```python
from build123d import *

# Parameters (mm, degrees)
CROQUIS1_R              = 1.5
SALIENTE_EXTRUIR1_DEPTH = 9


with BuildPart() as part:
    # Croquis1 → Saliente-Extruir1 (new body)
    with BuildSketch(Plane(origin=(0, 0, 0), x_dir=(1, 0, 0), z_dir=(0, 1, 0))):
        Polygon((7.75, 7.5), (26.5, 22.904273087), (26.5, 77.904273087), (26.5, 87.904273087), (41.5, 77.904273087), (41.5, 22.904273087), (22.75, 7.5), (22.75, -7.5), (7.75, -7.5), align=None)
        with Locations(Location((19.25, 4, 0), (0, 0, 270))):
            Circle(CROQUIS1_R, mode=Mode.SUBTRACT)
        with Locations(Location((19.25, -4, 0), (0, 0, 270))):
            Circle(CROQUIS1_R, mode=Mode.SUBTRACT)
        with Locations(Location((11.25, -4, 0), (0, 0, 270))):
            Circle(CROQUIS1_R, mode=Mode.SUBTRACT)
        with Locations(Location((11.25, 4, 0), (0, 0, 270))):
            Circle(CROQUIS1_R, mode=Mode.SUBTRACT)
    extrude(amount=SALIENTE_EXTRUIR1_DEPTH)


solid = part.part
```
Here's how the part is built. I have some questions about the finished solid (model axes, mm). A direction names the side the tool comes from. Round coordinates to 2 decimals unless told otherwise and drop trailing zeros. Order: outer loops, then holes, each group sorted by start corner. A loop starts at its lowest first (then second) coordinate and runs counter-clockwise, first axis right, second up. Notation, with made-up numbers: (10.25, 69.25) -> (49.25, 69.25) arc R21 ccw to (49.25, 75.25) -> close; hole circle Ø6 at (59, -11). An arc over 180 degrees is marked (long way). Use a Markdown table: item, result. Add a question column.
(1) I need wall thicknesses on line 1 along X through (y, z) = (4, -4); line 2 along Z through (x, y) = (20, 2.25); line 3 along X through (y, z) = (2, -71). Which ranges of each line are inside material? Lowest first, please.
(2) For faces 1 (the face through (41.5, 4, -51)), 2 (the face through (22.75, 4, 0)), 3 (the face through (26.5, 4, -56)), which set-ups out of +Z, -Z, +X, -X, +Y, -Y let a thin tool reach every point of the face, with its end or its side?
(3) Suppose I cut it at A-A, the plane z = -4. Please give me the cut outline in (x, y), and give its area (3 significant figures).
(4) For pin 1 Ø1.5 at (y, z) = (2, -64.5) entering from -X; pin 2 Ø2.5 at (y, z) = (6.5, -2.5) entering from +X, each with a flat end and sliding along its axis, tell me the tip position at first contact or that it passes through.
(5) Suppose I cut it at B-B, the plane y = 3.5. Please give me the cut outline in (x, z).
(6) Suppose I cut it at D-D, the plane z = -43. Please give me the cut outline in (x, y).
(7) Suppose I cut it at C-C, the plane x = 19.25. Please give me the cut outline in (y, z), and give its area (3 significant figures).
(8) If we mould it in two halves opening along Z, with no side actions, what happens to faces 4 (the face through (20.515, 4.437, -3.194)), 5 (the face through (15, 4, 7.5)), 6 (the face through (29, 0, -41))? For each: released by +Z, released by -Z, zero draft, split by the parting line, or undercut.
Verdict:
| question | item | result |
|---|---|---|
| 1 | line 1 | 7.75 to 9.75, 12.75 to 17.75, 20.75 to 22.75 |
| 1 | line 2 | -17.56 to -5.3, -2.7 to 2.7, 5.3 to 7.5 |
| 1 | line 3 | 26.5 to 41.5 |
| 2 | face 1 | +Z, -Z, +X, +Y, -Y |
| 2 | face 2 | +Z, +X, +Y, -Y |
| 2 | face 3 | -Z, -X, +Y, -Y |
| 3 | outline | (7.75, 0) -> (9.75, 0) -> (9.75, 9) -> (7.75, 9) -> close; (12.75, 0) -> (17.75, 0) -> (17.75, 9) -> (12.75, 9) -> close; (20.75, 0) -> (22.75, 0) -> (22.75, 9) -> (20.75, 9) -> close |
| 3 | area | 81.0 mm2 |
| 4 | pin 1 | x = 26.5 |
| 4 | pin 2 | x = 22.75 |
| 5 | outline | (7.75, -7.5) -> (26.5, -22.9) -> (26.5, -87.9) -> (41.5, -77.9) -> (41.5, -22.9) -> (22.75, -7.5) -> (22.75, 7.5) -> (7.75, 7.5) -> close; hole circle Ø3 at (11.25, -4); hole circle Ø3 at (11.25, 4); hole circle Ø3 at (19.25, -4); hole circle Ø3 at (19.25, 4) |
| 6 | outline | (26.5, 0) -> (41.5, 0) -> (41.5, 9) -> (26.5, 9) -> close |
| 7 | outline | (0, -16.95) -> (9, -16.95) -> (9, -5.5) -> (0, -5.5) -> close; (0, -2.5) -> (9, -2.5) -> (9, 2.5) -> (0, 2.5) -> close; (0, 5.5) -> (9, 5.5) -> (9, 7.5) -> (0, 7.5) -> close |
| 7 | area | 166 mm2 |
| 8 | face 4 | undercut |
| 8 | face 5 | released by +Z |
| 8 | face 6 | zero draft |
